Here's how the part is built. I have some questions about the finished solid (model axes, mm). Give positions to 0.01 mm unless a question says otherwise; leave off trailing zeros. Write each loop counter-clockwise with the first axis right and the second up, starting at its lowest first coordinate (ties: lowest second). Pieces come first, ordered by that corner, then holes. Notation, with made-up numbers: (-39, 47.5) - (-20, 47.5) arc R16 ccw to (-20, 61.5) - close; hole circle Ø4 at (8, 32). An arc over 180 degrees is marked (long way). Use a Markdown table: item, result.
Autodesk Inventor part; units mm, degrees
ref_plane "YZ Plane" through (0, 0, 0) normal (1, 0, 0) x (0, 1, 0)
ref_plane "XZ Plane" through (0, 0, 0) normal (0, 1, 0) x (-1, 0, 0)
ref_plane "XY Plane" through (0, 0, 0) normal (0, 0, 1) x (1, 0, 0)
sketch "スケッチ1" plane through (0, 0, 0) normal (0, 0, 1) x (1, 0, 0)
  line L0 (0, 0) -> (135, 0)
  line L1 (135, 0) -> (135, 50)
  line L2 (135, 50) -> (0, 50)
  line L3 (0, 50) -> (0, 0)
  dimension "d0" = 135
  dimension "d1" = 50
extrude "押し出し1" add sketch "スケッチ1" along normal blind 4
sketch "スケッチ2" plane through (0, 0, 4) normal (0, 0, 1) x (1, 0, 0)
  line L0 (5, 40.2) -> (11.3, 40.2)
  line L1 (11.3, 40.2) -> (11.3, 29.9)
  line L2 (11.3, 29.9) -> (5, 29.9)
  line L3 (5, 29.9) -> (5, 40.2)
  line L4 (135, 50) -> (0, 50)
  line L5 (0, 50) -> (0, 0)
  line L6 (0, 25) -> (135, 25)
  line L7 (135, 0) -> (135, 50)
  line L8 (67.5, 50) -> (67.5, 0)
  line L9 (0, 0) -> (135, 0)
  line L10 (5, 9.8) -> (11.3, 9.8)
  line L11 (11.3, 9.8) -> (11.3, 20.1)
  line L12 (11.3, 20.1) -> (5, 20.1)
  line L13 (5, 20.1) -> (5, 9.8)
  line L14 (130, 40.2) -> (123.7, 40.2)
  line L15 (123.7, 40.2) -> (123.7, 29.9)
  line L16 (123.7, 29.9) -> (130, 29.9)
  line L17 (130, 29.9) -> (130, 40.2)
  line L18 (135, 25) -> (0, 25)
  line L19 (130, 9.8) -> (123.7, 9.8)
  line L20 (123.7, 9.8) -> (123.7, 20.1)
  line L21 (123.7, 20.1) -> (130, 20.1)
  line L22 (130, 20.1) -> (130, 9.8)
  dimension "d4" = 6.3
  dimension "d5" = 10.3
  dimension "d6" = 9.8
  dimension "d7" = 5
extrude "押し出し2" cut sketch "スケッチ2" against normal blind 10 contours L0 L1 L2 L3 | L13 L12 L11 L10 | L17 L16 L15 L14 | L19 L20 L21 L22
sketch "スケッチ3" plane through (0, 0, 4) normal (0, 0, 1) x (1, 0, 0)
  line L0 (11.3, 29.9) -> (5, 29.9)
  line L1 (0, 50) -> (0, 0)
  line L2 (135, 50) -> (0, 50)
  line L3 (67.5, 50) -> (67.5, 0)
  line L4 (0, 0) -> (135, 0)
  point P0 (8.15, 25)
  point P1 (126.85, 25)
  dimension "d10" = 4.9
  dimension "d11" = 8.15
hole "穴1" at (8.15, 25, 4) at (126.85, 25, 4) direction (0, 0, -1) diameter 3.6 depth 4.5
fillet "フィレット1" radius 2 4 edges at (0, 25, 4) (0, 25, 0) (135, 25, 4) (135, 25, 0)
properties part number "menteB"
Item 1: I need wall thicknesses on line 1 along Y through (x, z) = (126.85, 2.7); line 2 along Y through (x, z) = (125, 0.55); line 3 along X through (y, z) = (25, 3.15). Which ranges of each line are inside material? Lowest first, please. Write a range as [from, to].
Values:
| item | result |
|---|---|
| line 1 | y = [0, 9.8], [20.1, 23.2], [26.8, 29.9], [40.2, 50] |
| line 2 | y = [0, 9.8], [20.1, 29.9], [40.2, 50] |
| line 3 | x = [0.36, 6.35], [9.95, 125.05], [128.65, 134.64] |
Item 2: If we section it at A-A, the plane x = 126.85: Write out the boundary of the cut face in (y, z), plus the area to 3 significant figures.
Values:
| item | result |
|---|---|
| outline | (0, 0) - (9.8, 0) - (9.8, 4) - (0, 4) - close; (20.1, 0) - (23.2, 0) - (23.2, 4) - (20.1, 4) - close; (26.8, 0) - (29.9, 0) - (29.9, 4) - (26.8, 4) - close; (40.2, 0) - (50, 0) - (50, 4) - (40.2, 4) - close |
| area | 103 mm2 |
Item 3: If we section it at B-B, the plane y = 25: Count the separate pieces of the cut face and the enclosed holes in it, plus the area to 3 significant figures.
Values:
| item | result |
|---|---|
| separate pieces | 3 |
| enclosed holes | 0 |
| area | 508 mm2 |
Item 4: Thinking about a two-plate mould opening in Y: for faces 1 (the flat face through (67, 0, 2)), 2 (the flat face through (130, 35, 2)), 3 (the flat face through (67, 25, 4)), which applies, +Y half, -Y half, draft (parallel to the pull), parting line (faces both ways), or undercut?
Values:
| item | result |
|---|---|
| face 1 | -Y half |
| face 2 | undercut |
| face 3 | draft |
